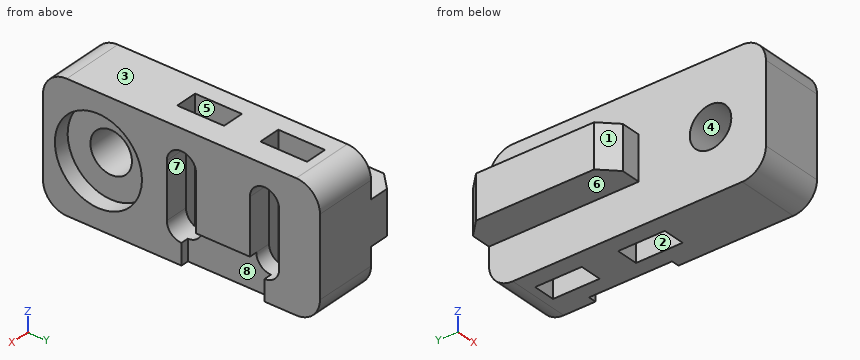
```python
from build123d import *

# Parameters (mm, degrees)
SKETCH1_W           = 16
SKETCH1_H           = 35
BOSS_EXTRUDE1_DEPTH = 8
SKETCH2_W           = 5.5
SKETCH2_H           = 18.925407089
BOSS_EXTRUDE2_DEPTH = 4.5
CHAMFER1_SIZE       = 2
CUT_EXTRUDE1_START  = -3
SKETCH7_W           = 16
SKETCH7_H           = 5.9
CUT_EXTRUDE1_DEPTH  = 2.8
CUT_EXTRUDE2_DEPTH  = 5
SKETCH9_W           = 4.5
SKETCH9_H           = 10.5
CUT_EXTRUDE3_DEPTH  = 1
FILLET7_R           = 3
SKETCH10_R          = 2.625
CUT_EXTRUDE4_DEPTH  = 20
SKETCH11_R          = 5.5
CUT_EXTRUDE5_DEPTH  = 2


with BuildPart() as part:
    # Sketch1 → Boss-Extrude1 (new body)
    with BuildSketch(Plane(origin=(0, 0, 0), x_dir=(0, 0, -1), z_dir=(1, 0, 0))):
        with Locations((-40.846556001, 15.41146402)):
            Rectangle(SKETCH1_W, SKETCH1_H)
    extrude(amount=BOSS_EXTRUDE1_DEPTH)

    # Sketch2 → Boss-Extrude2 (add)
    with BuildSketch(Plane.ZY):
        with Locations((40.846556001, 23.448760476)):
            Rectangle(SKETCH2_W, SKETCH2_H)
    extrude(amount=BOSS_EXTRUDE2_DEPTH)

    # Chamfer1
    chamfer1_edges = [part.edges().sort_by_distance(p)[0] for p in [
        (-4.5, 13.986056931, 40.846556001),
        (-4.5, 32.91146402, 40.846556001),
    ]]
    chamfer(chamfer1_edges, length=CHAMFER1_SIZE)

    # Sketch7 → Cut-Extrude1 (cut)
    with BuildSketch(Plane(origin=(8, 0, 0), x_dir=(0, 0, -1), z_dir=(1, 0, 0)).offset(CUT_EXTRUDE1_START)):
        with Locations((-40.846556001, 25.91146402)):
            Rectangle(SKETCH7_W, SKETCH7_H)
        with Locations((-40.846556001, 15.41146402)):
            Rectangle(SKETCH7_W, SKETCH7_H)
    extrude(amount=-CUT_EXTRUDE1_DEPTH, mode=Mode.SUBTRACT)

    # Sketch8 → Cut-Extrude2 (cut)
    with BuildSketch(Plane(origin=(8, 0, 0), x_dir=(0, 0, -1), z_dir=(1, 0, 0))):
        with BuildLine():
            Line((-44.346556001, 27.76146402), (-37.346556001, 27.76146402))
            ThreePointArc((-37.346556001, 27.76146402), (-35.496556001, 25.91146402), (-37.346556001, 24.06146402))
            Line((-37.346556001, 24.06146402), (-44.346556001, 24.06146402))
            ThreePointArc((-44.346556001, 24.06146402), (-46.196556001, 25.91146402), (-44.346556001, 27.76146402))
        make_face()
        with BuildLine():
            Line((-44.346556001, 17.26146402), (-37.346556001, 17.26146402))
            ThreePointArc((-37.346556001, 17.26146402), (-35.496556001, 15.41146402), (-37.346556001, 13.56146402))
            Line((-37.346556001, 13.56146402), (-44.346556001, 13.56146402))
            ThreePointArc((-44.346556001, 13.56146402), (-46.196556001, 15.41146402), (-44.346556001, 17.26146402))
        make_face()
    extrude(amount=-CUT_EXTRUDE2_DEPTH, mode=Mode.SUBTRACT)

    # Sketch9 → Cut-Extrude3 (cut)
    with BuildSketch(Plane(origin=(8, 0, 0), x_dir=(0, 0, -1), z_dir=(1, 0, 0))):
        with Locations((-35.096556001, 20.66146402)):
            Rectangle(SKETCH9_W, SKETCH9_H)
    extrude(amount=-CUT_EXTRUDE3_DEPTH, mode=Mode.SUBTRACT)

    # Fillet7
    fillet7_edges = [part.edges().sort_by_distance(p)[0] for p in [
        (4, 32.91146402, 32.846556001),
        (4, 32.91146402, 48.846556001),
        (4, -2.08853598, 48.846556001),
        (4, -2.08853598, 32.846556001),
    ]]
    fillet(fillet7_edges, radius=FILLET7_R)

    # Sketch10 → Cut-Extrude4 (cut)
    with BuildSketch(Plane(origin=(8, 0, 0), x_dir=(0, 0, -1), z_dir=(1, 0, 0))):
        with Locations((-40.846556001, 4.91146402)):
            Circle(SKETCH10_R)
    extrude(amount=-CUT_EXTRUDE4_DEPTH, mode=Mode.SUBTRACT)

    # Sketch11 → Cut-Extrude5 (cut)
    with BuildSketch(Plane(origin=(8, 0, 0), x_dir=(0, 0, -1), z_dir=(1, 0, 0))):
        with Locations((-40.846556001, 4.91146402)):
            Circle(SKETCH11_R)
    extrude(amount=-CUT_EXTRUDE5_DEPTH, mode=Mode.SUBTRACT)


solid = part.part
```
Source: CAD feature listing. Evaluate the final solid. Frame: model axes, mm. Face numbers are marked on the shaded views. A direction names the side the tool comes from. Round coordinates to 2 decimals unless told otherwise and drop trailing zeros. Order: outer loops, then holes, each group sorted by start corner. A loop starts at its lowest first (then second) coordinate and runs counter-clockwise, first axis right, second up. Notation, with made-up numbers: (-21, 12) -> (16, 12) arc R26 ccw to (16, 43) -> close; hole circle Ø11 at (-0.75, 23). An arc over 180 degrees is marked (long way). One line per item, written item: value. Start each with the question number.
Q1. Draft query along Y for the marked faces 1, 2 and 3. Return one class per face: pulls with the +Y half, pulls with the -Y half, needs draft (parallel to the pull), parting line crosses it, or undercut.
Q2. Access query for the marked faces 4, 5, 6, 7 and 8. Directions: +Z, -Z, +X, -X, +Y, -Y. A direction counts if a zero-diameter tool reaches every point of the face in a straight line with its end or side. Return the directions, or none.
Q3. Section query C-C (y = 4). Return the cut outline in (x, z).
Q4. Material intervals for probe 1 along Y at (x, z) = (3.75, 46.5); probe 2 along X at (y, z) = (12, 46); probe 3 along Z at (x, y) = (-2, 23.5), sorted ascending.
Q5. Section query D-D (y = 19.5). Return the cut outline in (x, z), plus the area to 3 significant figures.
Q6. Pin query (flat end, axial travel): pin 1 (0.8 mm diameter, centred on x = 7.5, y = 19.5, fed in from -Z); pin 2 (2 mm diameter, centred on x = -3.5, y = 26.5, fed in from -Z). Return the tip coordinate at first contact, or that it passes through.
Q7. Section query A-A (x = 2.75). Return the cut outline in (y, z) (3 decimals).
Findings below:
1. face 1: pulls with the -Y half
1. face 2: undercut
1. face 3: needs draft
2. face 4: +X, -X
2. face 5: +Z, -Z
2. face 6: -Z, -X, +Y, -Y
2. face 7: +X
2. face 8: -Z, +X
3. outline: (0, 32.85) -> (8, 32.85) -> (8, 35.42) -> (6, 35.42) -> (6, 38.38) -> (0, 38.38) -> close; (0, 43.31) -> (6, 43.31) -> (6, 46.27) -> (8, 46.27) -> (8, 48.85) -> (0, 48.85) -> close
4. probe 1: -2.02 to 12.46, 18.36 to 22.96, 28.86 to 32.84
4. probe 2: 0 to 8
4. probe 3: 38.1 to 43.6
5. outline: (-4.5, 38.1) -> (0, 38.1) -> (0, 32.85) -> (7, 32.85) -> (7, 37.35) -> (8, 37.35) -> (8, 48.85) -> (0, 48.85) -> (0, 43.6) -> (-4.5, 43.6) -> close
5. area: 148 mm²
6. pin 1: z = 37.35
6. pin 2: z = 38.1
7. outline: (-2.089, 35.847) arc R3 ccw to (0.911, 32.847) -> (12.461, 32.847) -> (12.461, 48.847) -> (0.911, 48.847) arc R3 ccw to (-2.089, 45.847) -> close; (18.361, 32.847) -> (22.961, 32.847) -> (22.961, 48.847) -> (18.361, 48.847) -> close; (28.861, 32.847) -> (29.911, 32.847) arc R3 ccw to (32.911, 35.847) -> (32.911, 45.847) arc R3 ccw to (29.911, 48.847) -> (28.861, 48.847) -> close; hole circle Ø5.25 at (4.911, 40.847)
